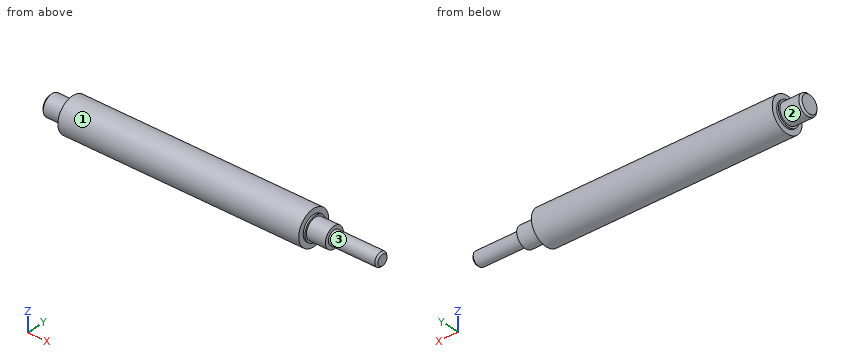
from build123d import *

# Parameters (mm, degrees)
CHAMFER1_SIZE = 0.5


with BuildPart() as part:
    # Sketch1 → Revolve1 (revolve)
    with BuildSketch(Plane.XY):
        Polygon((0, 0), (0, 3), (6, 3), (6, 3.5), (6.5, 3.5), (6.5, 5), (76.5, 5), (76.5, 3.5), (77, 3.5), (77, 3), (82.5, 3), (82.5, 2), (96.5, 2), (96.5, 0), align=None)
    revolve(axis=Axis((96.5, 0, 0), (-1, 0, 0)))

    # Chamfer1
    chamfer1_edges = [part.edges().sort_by_distance(p)[0] for p in [
        (0, -3, 0),
        (96.5, -2, 0),
    ]]
    chamfer(chamfer1_edges, length=CHAMFER1_SIZE)


solid = part.part
Part model, mm, in its own coordinate system. Face numbers are marked on the shaded views. A direction names the side the tool comes from. Round coordinates to 2 decimals unless told otherwise and drop trailing zeros. Order: outer loops, then holes, each group sorted by start corner. A loop starts at its lowest first (then second) coordinate and runs counter-clockwise, first axis right, second up. Notation, with made-up numbers: (-39.75, -39) -> (-11.75, -39) arc R19 cw to (-11.75, -18) -> close; hole circle Ø5 at (88.25, 54). An arc over 180 degrees is marked (long way). Put each result on its own line as item: value.
Q1. Pin check, flat tips, straight feed: pin 1 Ø3 at (x, z) = (57, 2) entering from +Y; pin 2 Ø5 at (x, y) = (66.5, 0.5) entering from -Z; pin 3 Ø2 at (x, z) = (60, -3) entering from -Y; pin 4 Ø2 at (y, z) = (1, -3.5) entering from +X. Stop position of each tip, or through.
From the geometry:
pin 1: stops at y = 4.97
pin 2: stops at z = -5
pin 3: stops at y = -4.58
pin 4: stops at x = 82.5
Q2. Wall check: line 1 (X direction, y = -2.25, z = -3.75); line 2 (Y direction, x = 18.5, z = 4); line 3 (X direction, y = -2, z = 1). Give the ranges that are in metal, low to high. Write a range as [from, to].
From the geometry:
line 1: x = [6.5, 76.5]
line 2: y = [-3, 3]
line 3: x = [0, 82.5]
Q3. Band-saw the part on A-A (y = 0). Give the cut face in (x, z).
From the geometry:
outline: (0, -2.5) -> (0.5, -3) -> (6, -3) -> (6, -3.5) -> (6.5, -3.5) -> (6.5, -5) -> (76.5, -5) -> (76.5, -3.5) -> (77, -3.5) -> (77, -3) -> (82.5, -3) -> (82.5, -2) -> (96, -2) -> (96.5, -1.5) -> (96.5, 1.5) -> (96, 2) -> (82.5, 2) -> (82.5, 3) -> (77, 3) -> (77, 3.5) -> (76.5, 3.5) -> (76.5, 5) -> (6.5, 5) -> (6.5, 3.5) -> (6, 3.5) -> (6, 3) -> (0.5, 3) -> (0, 2.5) -> close
Q4. Band-saw the part on C-C (x = 35.5). Give the cut face in (y, z), and give its area (3 significant figures).
From the geometry:
outline: circle Ø10 at (0, 0)
area: 78.5 mm2
Q5. Tool access for the marked faces 1, 2 and 3: list every direction of +Z, -Z, +X, -X, +Y, -Y with a clear straight run to the whole face (end or side of a thin tool).
From the geometry:
face 1: +X, -X
face 2: -X
face 3: +X
